For this review, take the finished solid that the model builds, in its own axes (mm). A direction names the side the tool comes from. Coordinates: 2 decimals unless noted, no trailing zeros. Loops run counter-clockwise (first coordinate to the right, second up) from the corner with the lowest first, then second, coordinate; pieces in that order, holes last. Notation, with made-up numbers: M 18.5,77 L 47.5,77 A18 ccw 47.5,92 Z; hole C -20.75,-17.5 d5. An arc over 180 degrees is marked long. Answer as a JSON object with one key per item and string values. Group by question number.
Item 1: Insertion check: pin 1 (5 mm diameter, centred on x = 135, y = -25, fed in from +Z). The pin has a flat end and moves straight along its axis. Give the tip position at first contact, or say it passes through.
Item 2: Wall thickness on L1, parallel to Y at x = 39, z = 2.35; L2, parallel to Y at x = 75.5, z = 1.2; L3, parallel to Y at x = 123, z = 1.8: over which ranges is each line inside the solid? List them lowest first. Write a range as from..to.
Item 3: Add section B-B (y = -44.5). State the section outline as (x, z) points, then the cut area to 3 significant figures.
Item 4: Add section A-A (x = 15). State the section outline as (y, z) points, then the cut area to 3 significant figures.
Item 5: Mouldability with a two-part tool opening along X and no side actions: class faces 1 (the face through (35, -72, 2)), 2 (the face through (0, -40, 1)), 3 (the face through (76, -68, 2)), 4 (the face through (76, -39, 0)) as +X half, -X half, draft (parallel to the pull), parting line (faces both ways), or undercut.
Item 6: Add section C-C (x = 31.5). State the section outline as (y, z) points.
Item 7: Tool access review of faces 5 (the face through (54.912, -58.158, 1.521)), 6 (the face through (3.01, -77.15, 1.48)): name each direction out of +Z, -Z, +X, -X, +Y, -Y from which nothing blocks a thin tool from reaching the whole face with its end or side.
Item 8: Add section D-D (y = -8). State the section outline as (x, z) points.
from build123d import *

# Parameters (mm, degrees)
SKETCH_1_R          = 2.1
EXTRUDE_1_DEPTH     = 3
SKETCH_2_R          = 2.1
CUT_EXTRUDE_1_DEPTH = 3
SKETCH_3_R          = 7.5
CUT_EXTRUDE_2_DEPTH = 3


with BuildPart() as part:
    # 草图1 → 凸台-拉伸1 (new body)
    with BuildSketch(Plane.XY):
        with BuildLine():
            Line((10, 0), (140, 0))
            ThreePointArc((140, 0), (147.071067812, -2.928932188), (150, -10))
            Line((150, -10), (150, -70))
            ThreePointArc((150, -70), (147.071067812, -77.071067812), (140, -80))
            Line((140, -80), (10, -80))
            ThreePointArc((10, -80), (2.928932188, -77.071067812), (0, -70))
            Line((0, -70), (0, -10))
            ThreePointArc((0, -10), (2.928932188, -2.928932188), (10, 0))
        make_face()
        with Locations((8, -8)):
            Circle(SKETCH_1_R, mode=Mode.SUBTRACT)
        with Locations((8, -72)):
            Circle(SKETCH_1_R, mode=Mode.SUBTRACT)
        with Locations((142, -72)):
            Circle(SKETCH_1_R, mode=Mode.SUBTRACT)
        with Locations((142, -8)):
            Circle(SKETCH_1_R, mode=Mode.SUBTRACT)
    extrude(amount=EXTRUDE_1_DEPTH)

    # 草图2 → 切除-拉伸1 (cut)
    with BuildSketch(Plane.XY.offset(3)):
        with Locations((15, -25)):
            Circle(SKETCH_2_R)
        with Locations((39, -25)):
            Circle(SKETCH_2_R)
        with Locations((39, -55)):
            Circle(SKETCH_2_R)
        with Locations((15, -55)):
            Circle(SKETCH_2_R)
        with Locations(Location((111, -55, 0), (0, 0, 180))):
            Circle(SKETCH_2_R)
        with Locations(Location((111, -25, 0), (0, 0, 180))):
            Circle(SKETCH_2_R)
        with Locations(Location((135, -25, 0), (0, 0, 180))):
            Circle(SKETCH_2_R)
        with Locations(Location((135, -55, 0), (0, 0, 180))):
            Circle(SKETCH_2_R)
    extrude(amount=-CUT_EXTRUDE_1_DEPTH, mode=Mode.SUBTRACT)

    # 草图3 → 切除-拉伸2 (cut)
    with BuildSketch(Plane.XY.offset(3)):
        with Locations((27, -40)):
            Circle(SKETCH_3_R)
        with Locations(Location((123, -40, 0), (0, 0, 180))):
            Circle(SKETCH_3_R)
        with BuildLine():
            Line((39, -4), (111, -4))
            ThreePointArc((111, -4), (115, -8), (111, -12))
            Line((111, -12), (39, -12))
            ThreePointArc((39, -12), (35, -8), (39, -4))
        make_face()
        with BuildLine():
            Line((39, -76), (111, -76))
            ThreePointArc((111, -76), (115, -72), (111, -68))
            Line((111, -68), (39, -68))
            ThreePointArc((39, -68), (35, -72), (39, -76))
        make_face()
        with BuildLine():
            Line((65.743091516, -20.242227956), (52.243091516, -32.242227956))
            ThreePointArc((52.243091516, -32.242227956), (48.007772044, -31.993091516), (48.256908484, -27.757772044))
            Line((48.256908484, -27.757772044), (61.756908484, -15.757772044))
            ThreePointArc((61.756908484, -15.757772044), (65.992227956, -16.006908484), (65.743091516, -20.242227956))
        make_face()
        with BuildLine():
            Line((65.743091516, -59.757772044), (52.243091516, -47.757772044))
            ThreePointArc((52.243091516, -47.757772044), (48.007772044, -48.006908484), (48.256908484, -52.242227956))
            Line((48.256908484, -52.242227956), (61.756908484, -64.242227956))
            ThreePointArc((61.756908484, -64.242227956), (65.992227956, -63.993091516), (65.743091516, -59.757772044))
        make_face()
        with BuildLine():
            Line((84.256908484, -20.242227956), (97.756908484, -32.242227956))
            ThreePointArc((97.756908484, -32.242227956), (101.992227956, -31.993091516), (101.743091516, -27.757772044))
            Line((101.743091516, -27.757772044), (88.243091516, -15.757772044))
            ThreePointArc((88.243091516, -15.757772044), (84.007772044, -16.006908484), (84.256908484, -20.242227956))
        make_face()
        with BuildLine():
            Line((84.256908484, -59.757772044), (97.756908484, -47.757772044))
            ThreePointArc((97.756908484, -47.757772044), (101.992227956, -48.006908484), (101.743091516, -52.242227956))
            Line((101.743091516, -52.242227956), (88.243091516, -64.242227956))
            ThreePointArc((88.243091516, -64.242227956), (84.007772044, -63.993091516), (84.256908484, -59.757772044))
        make_face()
    extrude(amount=-CUT_EXTRUDE_2_DEPTH, mode=Mode.SUBTRACT)


solid = part.part
From the geometry:
{
 "1": {"pin 1": "stops at z = 3"},
 "2": {"L1": "y = -80..-76, -68..-57.1, -52.9..-27.1, -22.9..-12, -4..0", "L2": "y = -80..-76, -68..-12, -4..0", "L3": "y = -80..-47.5, -32.5..0"},
 "3": {"outline": "M 0,0 L 21,0 L 21,3 L 0,3 Z; M 33,0 L 117,0 L 117,3 L 33,3 Z; M 129,0 L 150,0 L 150,3 L 129,3 Z", "area": "378 mm²"},
 "4": {"outline": "M -80,0 L -57.1,0 L -57.1,3 L -80,3 Z; M -52.9,0 L -27.1,0 L -27.1,3 L -52.9,3 Z; M -22.9,0 L 0,0 L 0,3 L -22.9,3 Z", "area": "215 mm²"},
 "5": {"face 1": "undercut", "face 2": "-X half", "face 3": "undercut", "face 4": "draft"},
 "6": {"outline": "M -80,0 L -46,0 L -46,3 L -80,3 Z; M -34,0 L 0,0 L 0,3 L -34,3 Z"},
 "7": {"face 5": "+Z, -Z", "face 6": "+Z, -Z, -X, -Y"},
 "8": {"outline": "M 0.2,0 L 5.9,0 L 5.9,3 L 0.2,3 Z; M 10.1,0 L 35,0 L 35,3 L 10.1,3 Z; M 115,0 L 139.9,0 L 139.9,3 L 115,3 Z; M 144.1,0 L 149.8,0 L 149.8,3 L 144.1,3 Z"}
}
